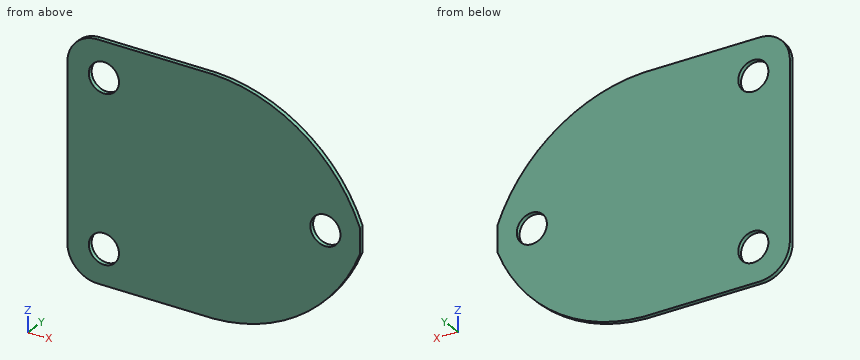
from build123d import *

# Parameters (mm, degrees)
F0_W     = 107.95
F0_H     = 86.0425
F1_DEPTH = 1.5875
F2_R     = 11.0998
F3_R     = 5.55625
F4_DEPTH = 1.5885
F6_DEPTH = 1.5885


with BuildPart() as f1:
    # F0 (on Front) → F1 (new body)
    with BuildSketch(Plane.XZ):
        Rectangle(F0_W, F0_H)
    extrude(amount=F1_DEPTH)

    # F2
    f2_edges = [f1.edges().sort_by_distance(p)[0] for p in [
        (-53.975, -0.79375, 43.02125),
        (-53.975, -0.79375, -43.02125),
    ]]
    fillet(f2_edges, radius=F2_R)

    # F3 (on Front) → F4 (cut, through all)
    with BuildSketch(Plane.XZ):
        with Locations((-40.4876, 30.1625)):
            Circle(F3_R)
        with Locations((-40.4876, -30.1625)):
            Circle(F3_R)
        with Locations((41.2496, 0)):
            Circle(F3_R)
    extrude(amount=F4_DEPTH, mode=Mode.SUBTRACT)

    # F5 (on Front) → F6 (cut, through all)
    with BuildSketch(Plane.XZ):
        with BuildLine():
            ThreePointArc((0, 43.02125), (34.718835, 30.470606), (55.5625, 0))
            ThreePointArc((55.5625, 0), (34.718835, -30.470606), (0, -43.02125))
            Line((0, -43.02125), (73.436641, -43.02125))
            Line((73.436641, -43.02125), (73.436641, 43.02125))
            Line((73.436641, 43.02125), (0, 43.02125))
        make_face()
    extrude(amount=F6_DEPTH, mode=Mode.SUBTRACT)


solid = f1.part
Here's how the part is built. I have some questions about the finished solid (model axes, mm). Round coordinates to 2 decimals unless told otherwise and drop trailing zeros. Loops run counter-clockwise (first coordinate to the right, second up) from the corner with the lowest first, then second, coordinate; pieces in that order, holes last. Notation, with made-up numbers: (68, 22.5) - (73, 22.5) arc R19 cw to (73, 31.5) - close; hole circle Ø4 at (1.5, 20). An arc over 180 degrees is marked (long way). One line per question, with ' | ' between items. Start each with the question number.
Q1. Please list where these lines run through material, in increasing order: line 1 (Z direction, x = -44.5, y = -0.55); line 2 (X direction, y = -1.4, z = -2) (3 decimals); line 3 (X direction, y = -0.8, z = 35). Write a range as [from, to].
Q2. I want a section at C-C (z = 34). Write out the boundary of the cut face in (x, y), then the cut area to 3 significant figures.
Q3. I want a section at B-B (y = -0.7). Write out the boundary of the cut face in (x, z) (1 decimal).
Q4. I want a section at A-A (z = 0). Write out the boundary of the cut face in (x, y) (1 decimal).
Q5. I want a section at D-D (x = 19). Write out the boundary of the cut face in (y, z), then the cut area to 3 significant figures.
Response values:
1) line 1: z = [-42.9, -34.01], [-26.32, 26.32], [34.01, 42.9] | line 2: x = [-53.975, 36.066], [46.433, 53.975] | line 3: x = [-53.54, -43.22], [-37.75, 27.97]
2) outline: (-53.78, -1.59) - (-44.51, -1.59) - (-44.51, 0) - (-53.78, 0) - close; (-36.47, -1.59) - (29.64, -1.59) - (29.64, 0) - (-36.47, 0) - close | area: 120 mm²
3) outline: (-54, -31.9) arc R11.1 ccw to (-42.9, -43) - (0, -43) arc R60.1 ccw to (54, -4.7) - (54, 4.7) arc R60.1 ccw to (0, 43) - (-42.9, 43) arc R11.1 ccw to (-54, 31.9) - close; hole circle Ø11.1 at (-40.5, -30.2); hole circle Ø11.1 at (-40.5, 30.2); hole circle Ø11.1 at (41.2, 0)
4) outline: (-54, -1.6) - (35.7, -1.6) - (35.7, 0) - (-54, 0) - close; (46.8, -1.6) - (54, -1.6) - (54, 0) - (46.8, 0) - close
5) outline: (-1.59, -39.24) - (0, -39.24) - (0, 39.24) - (-1.59, 39.24) - close | area: 125 mm²
